Input: part model. Units: mm. Frame: model coordinates. A direction names the side the tool comes from. Give positions to 0.01 mm unless a question says otherwise; leave off trailing zeros. Loops run counter-clockwise (first coordinate to the right, second up) from the corner with the lowest first, then second, coordinate; pieces in that order, holes last.
from build123d import *

# Parameters (mm, degrees)
EXTRUDE_1_DEPTH = 5


with BuildPart() as part:
    # Эскиз1 → Вытянуть1 (new body)
    with BuildSketch(Plane.XY):
        with BuildLine():
            Line((51.051218407, 63.479620652), (51.051218407, 85.650578056))
            ThreePointArc((51.051218407, 85.650578056), (29.802221193, 107.884883156), (-0.253175823, 114.408480022))
            ThreePointArc((-0.253175823, 114.408480022), (-29.956404055, 107.707451089), (-50.948781593, 85.650578205))
            Line((-50.948781593, 85.650578205), (-50.948781593, 63.479620652))
            ThreePointArc((-50.948781593, 63.479620652), (-49.676003697, 55.151129839), (-46.113662299, 47.516115329))
            ThreePointArc((-46.113662299, 47.516115329), (-43.24429549, 44.636868096), (-39.466032041, 43.137516297))
            ThreePointArc((-39.466032041, 43.137516297), (-27.599168456, 36.303107276), (-22.910878505, 23.436424124))
            Line((-22.910878505, 23.436424124), (-22.910878505, -29.232372122))
            Line((-22.910878505, -29.232372122), (22.801652741, -29.232372122))
            Line((22.801652741, -29.232372122), (22.801652741, 23.436424124))
            ThreePointArc((22.801652741, 23.436424124), (27.504627406, 36.320562274), (39.401754329, 43.145322895))
            ThreePointArc((39.401754329, 43.145322895), (43.142841115, 44.60959187), (46.005754814, 47.428020354))
            ThreePointArc((46.005754814, 47.428020354), (49.685829012, 55.090035656), (51.051218407, 63.479620652))
        make_face()
    extrude(amount=EXTRUDE_1_DEPTH)


solid = part.part
(1) Cut plane B-B (y = 18). Return the cut outline in (x, z).
Values follow:
outline: (-22.91, 0) - (22.8, 0) - (22.8, 5) - (-22.91, 5) - close
(2) Reachability of faces 1 (the flat face through (-1, 60, 0)), 2 (the flat face through (22.802, -3, 2)), 3 (the flat face through (-22.911, -3, 2)) from +Z, -Z, +X, -X, +Y, -Y: full face, straight path, thin tool, end or side. Return the list, or none.
Values follow:
face 1: -Z, +X, -X, +Y, -Y
face 2: +Z, -Z, +X, -Y
face 3: +Z, -Z, -X, -Y
(3) Cut plane C-C (x = -32). Return the cut outline in (y, z), and give its area (3 significant figures).
Values follow:
outline: (40.2, 0) - (106.49, 0) - (106.49, 5) - (40.2, 5) - close
area: 331 mm2
(4) Pin query (flat end, axial travel): pin 1 Ø1.5 at (y, z) = (46, 2.5) entering from -X; pin 2 Ø3 at (y, z) = (1, 3) entering from -X; pin 3 Ø3 at (x, z) = (-8.5, 1.5) entering from +Y. Return the tip coordinate at first contact, or that it passes through.
Values follow:
pin 1: stops at x = -45.56
pin 2: stops at x = -22.91
pin 3: stops at y = 114.46
(5) Cut plane A-A (z = 2.8). Return the cut outline in (x, y), and give its area (3 significant figures).
Values follow:
outline: (-50.95, 63.48) arc R29.67 ccw to (-46.11, 47.52) arc R10 ccw to (-39.47, 43.14) arc R20 cw to (-22.91, 23.44) - (-22.91, -29.23) - (22.8, -29.23) - (22.8, 23.44) arc R20 cw to (39.4, 43.15) arc R10 ccw to (46.01, 47.43) arc R29.78 ccw to (51.05, 63.48) - (51.05, 85.65) arc R52.52 ccw to (-0.25, 114.41) arc R52.52 ccw to (-50.95, 85.65) - close
area: 9,870 mm2
(6) Ray query, probe 1 along X at (y, z) = (13, 4.6); probe 2 along Y at (x, z) = (-30, 1); probe 3 along X at (y, z) = (105.5, 2.65). Return the intervals inside material, ascending.
Values follow:
probe 1: x = -22.91 to 22.8
probe 2: y = 38.71 to 107.68
probe 3: x = -33.51 to 33.66
